For this review, take the finished solid that the model builds, in its own axes (mm). A direction names the side the tool comes from. Coordinates: 2 decimals unless noted, no trailing zeros. Loops run counter-clockwise (first coordinate to the right, second up) from the corner with the lowest first, then second, coordinate; pieces in that order, holes last.
1. Take a section at A-A, the plane y = 0. State the section outline as (x, z) points.
2. Take a section at B-B, the plane z = 40. State the section outline as (x, y) points, then the cut area to 3 significant figures.
3. Clearance check with flat-ended pins moving along their axes: P1, Ø1.5, axis at y = -1.5, z = 13.5, coming from the +X side; P2, Ø8.5, axis at y = 0, z = 48.93, coming from the +X side; P3, Ø10, axis at x = 6, z = 13.5, coming from the +Y side. State where each tip first meets the part, or that it passes through.
4. To check wall thickness, follow probe 1 along Z at (x, y) = (-13, 0); probe 2 along Z at (x, y) = (8.5, 0); probe 3 along Z at (x, y) = (57, 30.5). State the ranges of each line that lie inside material, in increasing order.
5. Take a section at D-D, the plane x = -6.5. State the section outline as (y, z) points (3 decimals), then the cut area to 3 significant figures.
6. Machinability: for faces 1 (the face through (-12.524, -0.688, 46.115)), 2 (the face through (24.227, 7.629, 44.272)), 3 (the face through (12.522, -0.688, 52.026)), which of the approach directions +Z, -Z, +X, -X, +Y, -Y give a long, thin tool a straight path to every point of the face, cutting with its end or side? Answer none if there is none.
7. Take a section at C-C, the plane x = 52.5. State the section outline as (y, z) points, then the cut area to 3 significant figures.
```python
from build123d import *

# Parameters (mm, degrees)
F0_W     = 152.4
F0_H     = 152.4
F1_DEPTH = 6.35
F2_R     = 38.1
F3_DEPTH = 25.4
F4_R     = 25.4
F5_DEPTH = 25.4
F7_D     = 6.35
F7_DEPTH = 76.201
F9_D     = 6.35
F9_DEPTH = 76.201


with BuildPart() as f1:
    # F0 (on Top) → F1 (new body)
    with BuildSketch(Plane.XY):
        Rectangle(F0_W, F0_H)
    extrude(amount=F1_DEPTH)

    # F2 (on face) → F3 (join)
    with BuildSketch(Plane.XY.offset(6.35)):
        Circle(F2_R)
    extrude(amount=F3_DEPTH)

    # F4 (on face) → F5 (join)
    with BuildSketch(Plane.XY.offset(31.75)):
        Circle(F4_R)
    extrude(amount=F5_DEPTH)

    # F7 (through all, one way)
    with BuildSketch(Plane(origin=(0, 0, 0), x_dir=(0, 1, 0), z_dir=(-1, 0, 0))):
        with Locations((0, -48.9269793034)):
            Circle(F7_D / 2)
    extrude(amount=-F7_DEPTH, mode=Mode.SUBTRACT)

    # F9 (through all, one way)
    with BuildSketch(Plane.YZ):
        with Locations((0, 49.2147840559)):
            Circle(F9_D / 2)
    extrude(amount=-F9_DEPTH, mode=Mode.SUBTRACT)


solid = f1.part
```
Results list:
1. outline: (-76.2, 0) - (76.2, 0) - (76.2, 6.35) - (38.1, 6.35) - (38.1, 31.75) - (25.4, 31.75) - (25.4, 45.75) - (0, 45.75) - (0, 46.04) - (-25.4, 46.04) - (-25.4, 31.75) - (-38.1, 31.75) - (-38.1, 6.35) - (-76.2, 6.35) - close; (-25.4, 52.39) - (0, 52.39) - (0, 52.1) - (25.4, 52.1) - (25.4, 57.15) - (-25.4, 57.15) - close
2. outline: circle Ø50.8 at (0, 0)
2. area: 2,030 mm2
3. P1: stops at x = 38.09
3. P2: stops at x = 25.4
3. P3: stops at y = 38.09
4. probe 1: z = 0 to 46.04, 52.39 to 57.15
4. probe 2: z = 0 to 45.75, 52.1 to 57.15
4. probe 3: z = 0 to 6.35
5. outline: (-76.2, 0) - (76.2, 0) - (76.2, 6.35) - (37.541, 6.35) - (37.541, 31.75) - (24.554, 31.75) - (24.554, 57.15) - (-24.554, 57.15) - (-24.554, 31.75) - (-37.541, 31.75) - (-37.541, 6.35) - (-76.2, 6.35) - close; hole circle Ø6.35 at (0, 49.215)
5. area: 4,090 mm2
6. face 1: -X
6. face 2: +Z
6. face 3: +X
7. outline: (-76.2, 0) - (76.2, 0) - (76.2, 6.35) - (-76.2, 6.35) - close
7. area: 968 mm2
